Part model, mm, in its own coordinate system. Face numbers are marked on the shaded views. A direction names the side the tool comes from. Give positions to 0.01 mm unless a question says otherwise; leave off trailing zeros. Order: outer loops, then holes, each group sorted by start corner. A loop starts at its lowest first (then second) coordinate and runs counter-clockwise, first axis right, second up. Notation, with made-up numbers: (-10, -3) - (45, -3) arc R26 cw to (45, 19) - close; hole circle Ø4 at (89.25, -21.75). An arc over 180 degrees is marked (long way). Use one line per item in the form item = value. Start each with the question number.
1. Band-saw the part on C-C, the plane y = -102. List the corners of the cut face in (x, z).
2. Band-saw the part on D-D, the plane z = -6. List the corners of the cut face in (x, y).
3. Band-saw the part on A-A, the plane x = 0. List the corners of the cut face in (y, z).
4. Tool access for the marked faces 1 and 2: list every direction of +Z, -Z, +X, -X, +Y, -Y with a clear straight run to the whole face (end or side of a thin tool).
5. Band-saw the part on B-B, the plane z = 0. List the corners of the cut face in (x, y).
6. Pin check, flat tips, straight feed: P1, Ø2, axis at x = -5.5, y = -45.5, coming from the +Z side; P2, Ø1, axis at y = -72.5, z = -4.5, coming from the -X side; P3, Ø5, axis at y = -47, z = 2.5, coming from the +X side; P4, Ø8, axis at x = -4, z = 2.5, coming from the +Y side. Stop position of each tip, or through.
7. Drill centre lines: line 1 (Y direction, x = 0, z = 2.25); line 2 (Y direction, x = 4.5, z = 2.25); line 3 (X direction, y = -101, z = -2.75). Where is each one in solid material? Low to high.
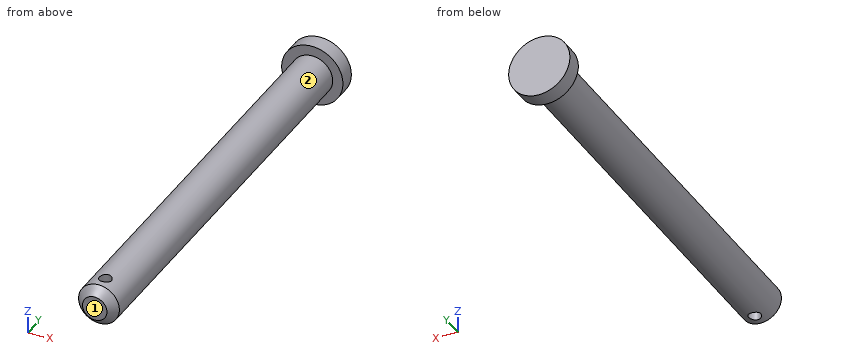
from build123d import *

# Parameters (mm, degrees)
F0_R     = 7.5
F1_DEPTH = 4
F2_R     = 5
F3_DEPTH = 103
F4_R     = 1.5
F5_DEPTH = 12.5
F6_SIZE  = 2


with BuildPart() as f1:
    # F0 (on Front) → F1 (new body)
    with BuildSketch(Plane.XZ):
        Circle(F0_R)
    extrude(amount=F1_DEPTH)

    # F2 (on face) → F3 (join)
    with BuildSketch(Plane.XZ.offset(4)):
        Circle(F2_R)
    extrude(amount=F3_DEPTH)

    # F4 (on Top) → F5 (cut, symmetric)
    with BuildSketch(Plane.XY):
        with Locations((0, -102)):
            Circle(F4_R)
    extrude(amount=F5_DEPTH, both=True, mode=Mode.SUBTRACT)

    # F6
    f6_edges = [f1.edges().sort_by_distance(p)[0] for p in [
        (-5, -107, 0),
    ]]
    chamfer(f6_edges, length=F6_SIZE)


solid = f1.part
From the geometry:
q1.outline = (-1.5, -4.77) - (-1.5, 4.77) arc R5 ccw to start; (1.5, -4.77) arc R5 ccw to (1.5, 4.77) - close
q2.outline = (-4.5, -4) - (4.5, -4) - (4.5, 0) - (-4.5, 0) - close
q3.outline = (-107, -3) - (-105, -5) - (-103.5, -5) - (-103.5, 5) - (-105, 5) - (-107, 3) - close; (-100.5, -5) - (-4, -5) - (-4, -7.5) - (0, -7.5) - (0, 7.5) - (-4, 7.5) - (-4, 5) - (-100.5, 5) - close
q4.face_1 = +Z, -Z, +X, -X, -Y
q4.face_2 = -Y
q5.outline = (-7.5, -4) - (-5, -4) - (-5, -105) - (-3, -107) - (3, -107) - (5, -105) - (5, -4) - (7.5, -4) - (7.5, 0) - (-7.5, 0) - close; hole circle Ø3 at (0, -102)
q6.P1 = 2.18
q6.P2 = -3
q6.P3 = 5
q6.P4 = 0
q7.line_1 = -107 to -103.5, -100.5 to 0
q7.line_2 = -4 to 0
q7.line_3 = -4.18 to -1.12, 1.12 to 4.18
